Input: part model. Units: mm. Frame: model coordinates. Face numbers are marked on the shaded views. A direction names the side the tool comes from. Round coordinates to 2 decimals unless told otherwise and drop trailing zeros. Loops run counter-clockwise (first coordinate to the right, second up) from the corner with the lowest first, then second, coordinate; pieces in that order, holes last. Notation, with made-up numbers: M 1,4.5 L 27,4.5 A30 cw 27,37.5 Z; hole C 55,66 d10. An arc over 180 degrees is marked long. Use one line per item in the form item = value. Start each with the question number.
Q1. Section query C-C, the plane x = -4.7. Output: boundary loops of the cut face in (y, z), and give its area (3 significant figures).
Q2. Section query A-A, the plane z = 14.5. Output: boundary loops of the cut face in (x, y).
Q3. Mould query, pull axis X, two halves, no side actions, for the marked faces 1, 2, 3 and 4. Classes: pulls with the +X half, pulls with the -X half, needs draft (parallel to the pull), parting line crosses it, or undercut.
Q4. Access query for the marked faces 5, 6 and 7. Directions: +Z, -Z, +X, -X, +Y, -Y. A direction counts if a zero-diameter tool reaches every point of the face in a straight line with its end or side. Return the directions, or none.
Q5. Section query D-D, the plane x = 16. Output: boundary loops of the cut face in (y, z), and give its area (3 significant figures).
Q6. Ray query, line 1 along Y through (x, z) = (13.5, 1.5); line 2 along Y through (x, z) = (14.5, 10); line 3 along Y through (x, z) = (-4.7, 2.05). Return the intervals inside material, ascending.
Q7. First-contact query: P1, Ø6, axis at y = 17, z = 13, coming from the +X side; P2, Ø4, axis at x = -4.7, y = 15, coming from the -Z side; P3, Ø9, axis at y = 16.5, z = 8.5, coming from the -X side. Flat tips, straight axial feed; report the tip coordinate or a pass-through.
Q8. Section query B-B, the plane y = 15. Output: boundary loops of the cut face in (x, z).
```python
from build123d import *

# Parameters (mm, degrees)
SKETCH1_W           = 26.3
SKETCH1_H           = 30.2
BOSS_EXTRUDE1_DEPTH = 21.5
CUT_EXTRUDE1_DEPTH  = 26
SKETCH3_W           = 44
SKETCH3_H           = 33
BOSS_EXTRUDE2_DEPTH = 3.1
CUT_EXTRUDE2_DEPTH  = 3.1
FILLET1_R           = 2
SKETCH5_W           = 28
SKETCH5_H           = 30.5
BOSS_EXTRUDE3_DEPTH = 1.4
FILLET2_R           = 2
SKETCH6_W           = 2
SKETCH6_H           = 2
CUT_EXTRUDE3_DEPTH  = 20
SKETCH7_R           = 1.6
CUT_EXTRUDE4_DEPTH  = 20


with BuildPart() as part:
    # Sketch1 → Boss-Extrude1 (new body)
    with BuildSketch(Plane.XY):
        with Locations((13.15, 15.1)):
            Rectangle(SKETCH1_W, SKETCH1_H)
    extrude(amount=BOSS_EXTRUDE1_DEPTH)

    # Sketch2 → Cut-Extrude1 (cut)
    with BuildSketch(Plane.XY.offset(21.5)):
        Polygon((0, 30.2), (0, 23.1), (5.95, 30.2), align=None)
        Polygon((20.35, 30.2), (26.3, 23.1), (26.3, 30.2), align=None)
    extrude(amount=-CUT_EXTRUDE1_DEPTH, mode=Mode.SUBTRACT)

    # Sketch3 → Boss-Extrude2 (add)
    with BuildSketch(Plane(origin=(0, 0, 0), x_dir=(-1, 0, 0), z_dir=(0, 0, -1))):
        with Locations((-13.3, 15)):
            Rectangle(SKETCH3_W, SKETCH3_H)
    extrude(amount=-BOSS_EXTRUDE2_DEPTH)

    # Sketch4 → Cut-Extrude2 (cut)
    with BuildSketch(Plane(origin=(0, 0, 0), x_dir=(-1, 0, 0), z_dir=(0, 0, -1))):
        Polygon((-35.3, 15), (-27.3, 31.5), (-35.3, 31.5), align=None)
        Polygon((8.7, 31.5), (0.7, 31.5), (8.7, 15), align=None)
        Polygon((8.7, -1.5), (8.7, 15), (0.7, -1.5), align=None)
        Polygon((-27.3, -1.5), (-35.3, 15), (-35.3, -1.5), align=None)
    extrude(amount=-CUT_EXTRUDE2_DEPTH, mode=Mode.SUBTRACT)

    # Fillet1
    fillet1_edges = [part.edges().sort_by_distance(p)[0] for p in [
        (27.3, 31.5, 1.55),
        (35.3, 15, 1.55),
        (-0.7, 31.5, 1.55),
        (-8.7, 15, 1.55),
        (-0.7, -1.5, 1.55),
        (27.3, -1.5, 1.55),
    ]]
    fillet(fillet1_edges, radius=FILLET1_R)

    # Sketch5 → Boss-Extrude3 (add)
    with BuildSketch(Plane(origin=(0, 0, 0), x_dir=(-1, 0, 0), z_dir=(0, 0, -1))):
        with Locations((-13.3, 15)):
            Rectangle(SKETCH5_W, SKETCH5_H)
    extrude(amount=BOSS_EXTRUDE3_DEPTH)

    # Fillet2
    fillet2_edges = [part.edges().sort_by_distance(p)[0] for p in [
        (-0.7, -0.25, -0.7),
        (-0.7, 30.25, -0.7),
        (27.3, 30.25, -0.7),
        (27.3, -0.25, -0.7),
    ]]
    fillet(fillet2_edges, radius=FILLET2_R)

    # Sketch6 → Cut-Extrude3 (cut)
    with BuildSketch(Plane(origin=(0, 0, -1.4), x_dir=(-1, 0, 0), z_dir=(0, 0, -1))):
        Polygon((-25.3, 24.25), (-25.3, 11.45), (-1.3, 11.45), (-1.3, 24.25), (-5.55, 28.45), (-21.05, 28.45), align=None)
        with Locations((-19.3, 18.45)):
            Rectangle(SKETCH6_W, SKETCH6_H, mode=Mode.SUBTRACT)
        with Locations((-7.3, 18.45)):
            Rectangle(SKETCH6_W, SKETCH6_H, mode=Mode.SUBTRACT)
        with Locations((-13.673670814, 23.25)):
            Rectangle(SKETCH6_W, SKETCH6_H, mode=Mode.SUBTRACT)
    extrude(amount=-CUT_EXTRUDE3_DEPTH, mode=Mode.SUBTRACT)

    # Sketch7 → Cut-Extrude4 (cut)
    with BuildSketch(Plane(origin=(0, 0, 0), x_dir=(-1, 0, 0), z_dir=(0, 0, -1))):
        with Locations((-31.3, 15)):
            Circle(SKETCH7_R)
        with Locations((4.7, 15)):
            Circle(SKETCH7_R)
    extrude(amount=-CUT_EXTRUDE4_DEPTH, mode=Mode.SUBTRACT)


solid = part.part
```
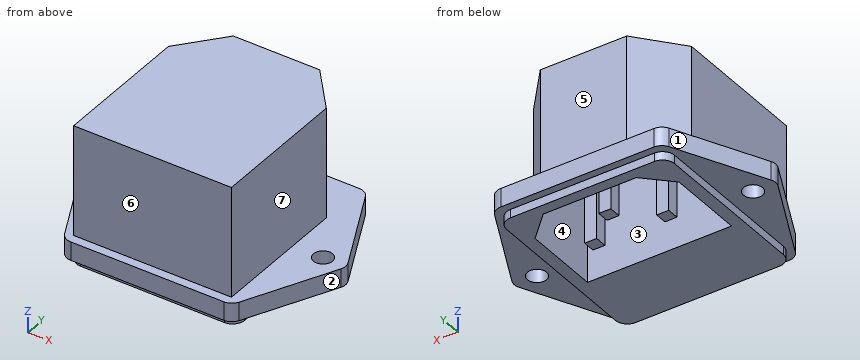
Results found:
q1.outline = M 6.75,0 L 13.4,0 L 13.4,3.1 L 6.75,3.1 Z; M 16.6,0 L 23.25,0 L 23.25,3.1 L 16.6,3.1 Z
q1.area = 41.2 mm²
q2.outline = M 0,0 L 26.3,0 L 26.3,23.1 L 20.35,30.2 L 5.95,30.2 L 0,23.1 Z; M 6.3,17.45 L 8.3,17.45 L 8.3,19.45 L 6.3,19.45 Z; M 12.67,22.25 L 14.67,22.25 L 14.67,24.25 L 12.67,24.25 Z; M 18.3,17.45 L 20.3,17.45 L 20.3,19.45 L 18.3,19.45 Z; hole M 1.3,11.45 L 25.3,11.45 L 25.3,24.25 L 21.05,28.45 L 5.55,28.45 L 1.3,24.25 Z
q3.face_1 = pulls with the -X half
q3.face_2 = pulls with the +X half
q3.face_3 = undercut
q3.face_4 = undercut
q4.face_5 = +Z, +X, -X, +Y
q4.face_6 = +Z, +X, -X, -Y
q4.face_7 = +Z, +X, +Y, -Y
q5.outline = M -1.5,0 L -0.25,0 L -0.25,-1.4 L 11.45,-1.4 L 11.45,18.6 L 28.45,18.6 L 28.45,-1.4 L 30.25,-1.4 L 30.25,0 L 31.5,0 L 31.5,3.1 L 30.2,3.1 L 30.2,21.5 L 0,21.5 L 0,3.1 L -1.5,3.1 Z
q5.area = 361 mm²
q6.line_1 = -1.5 to 11.45, 22.25 to 24.25, 28.45 to 31.5
q6.line_2 = 0 to 11.45, 22.25 to 24.25, 28.45 to 30.2
q6.line_3 = 6.75 to 13.4, 16.6 to 23.25
q7.P1 = 26.3
q7.P2 = 0
q7.P3 = 0
q8.outline = M -8.48,0 L -6.3,0 L -6.3,3.1 L -8.48,3.1 Z; M -3.1,0 L -0.7,0 L -0.7,-1.4 L 1.3,-1.4 L 1.3,18.6 L 25.3,18.6 L 25.3,-1.4 L 27.3,-1.4 L 27.3,0 L 29.7,0 L 29.7,3.1 L 26.3,3.1 L 26.3,21.5 L 0,21.5 L 0,3.1 L -3.1,3.1 Z; M 32.9,0 L 35.08,0 L 35.08,3.1 L 32.9,3.1 Z
